```python
from build123d import *

# Parameters (mm, degrees)
F1_DEPTH = 76.2
F2_R     = 6.35
F3_DEPTH = 76.2
F4_R     = 6.35
F5_DEPTH = 76.2


with BuildPart() as f1:
    # F0 (on Front) → F1 (new body)
    with BuildSketch(Plane.XZ):
        Polygon((-25.129344, 99.525434), (-75.929344, 99.525434), (-75.929344, -103.674566), (76.470656, -103.674566), (76.470656, -52.874566), (-25.129344, -52.874566), align=None)
    extrude(amount=F1_DEPTH)

    # F2 (on Right) → F3 (cut)
    with BuildSketch(Plane.YZ):
        with Locations((-38.1, 10.625434)):
            Circle(F2_R)
    extrude(amount=-F3_DEPTH, mode=Mode.SUBTRACT)

    # F4 (on Top) → F5 (cut)
    with BuildSketch(Plane.XY):
        with Locations((0, -38.1)):
            Circle(F4_R)
    extrude(amount=-F5_DEPTH, mode=Mode.SUBTRACT)


solid = f1.part
```
Build history of the part. All positions in model axes, mm. A direction names the side the tool comes from. Coordinates: 2 decimals unless noted, no trailing zeros. Order: outer loops, then holes, each group sorted by start corner. A loop starts at its lowest first (then second) coordinate and runs counter-clockwise, first axis right, second up. Notation, with made-up numbers: M 12,74 L 51,74 A13 cw 51,96 Z; hole C 46,48.5 d1. An arc over 180 degrees is marked long. One line per question, with ' | ' between items. Start each with the question number.
1. Cut at A-A (y = -38.1). Write the cut outline in (x, z), plus the area to 3 significant figures.
2. Wall check: line 1 along Z through (x, y) = (-50, -38); line 2 along X through (y, z) = (-38, -61); line 3 along Y through (x, z) = (0, -63.75). Give the ranges that are in metal, low to high. Write a range as [from, to].
3. Flat gauge pin, fed straight in: P1, Ø16.5, axis at x = 0, y = -38.1, coming from the +Z side. Where does the tip first touch, or does it go through?
4. Tool access for faces 1 (the face through (76.471, -38, -79)), 2 (the face through (6.057, -36.193, -64.374)), 3 (the face through (-25.129, -38, 22)): list every direction of +Z, -Z, +X, -X, +Y, -Y with a clear straight run to the whole face (end or side of a thin tool).
5. Cut at C-C (y = -28). Write the cut outline in (x, z).
6. Cut at D-D (z = 50). Write the cut outline in (x, y), plus the area to 3 significant figures.
7. Cut at B-B (x = 0). Write the cut outline in (y, z), plus the area to 3 significant figures.
8. Mould opens along Z. For faces 4 (the face through (-1, -38, -103.675)), 5 (the face through (-50, -38, 99.525)), 6 (the face through (-50.174, -32.043, 12.533)) say: +Z half, -Z half, draft (parallel to the pull), parting line (faces both ways), or undercut.
The answers:
1) outline: M -75.93,-103.67 L 76.47,-103.67 L 76.47,-52.87 L 6.35,-52.87 L 6.35,-76.2 L -6.35,-76.2 L -6.35,-52.87 L -25.13,-52.87 L -25.13,4.28 L -75.93,4.28 Z; M -75.93,16.98 L -25.13,16.98 L -25.13,99.53 L -75.93,99.53 Z | area: 14,500 mm2
2) line 1: z = [-103.67, 4.28], [16.97, 99.53] | line 2: x = [-75.93, -6.35], [6.35, 76.47] | line 3: y = [-76.2, -44.45], [-31.75, 0]
3) P1: stops at z = -52.87
4) face 1: +Z, -Z, +X, +Y, -Y | face 2: +Z | face 3: +Z, +X, +Y, -Y
5) outline: M -75.93,-103.67 L 76.47,-103.67 L 76.47,-52.87 L -25.13,-52.87 L -25.13,99.53 L -75.93,99.53 Z
6) outline: M -75.93,-76.2 L -25.13,-76.2 L -25.13,0 L -75.93,0 Z | area: 3,870 mm2
7) outline: M -76.2,-103.67 L 0,-103.67 L 0,-52.87 L -31.75,-52.87 L -31.75,-76.2 L -44.45,-76.2 L -44.45,-52.87 L -76.2,-52.87 Z | area: 3,570 mm2
8) face 4: -Z half | face 5: +Z half | face 6: undercut
